```python
from build123d import *

# Parameters (mm, degrees)
BOSS_EXTRUDE1_DEPTH = 12.7
SKETCH2_R           = 2.032
SKETCH2_R_2         = 3.96875
CUT_EXTRUDE1_DEPTH  = 93.361945119
SKETCH3_R           = 1.1303
CUT_EXTRUDE2_DEPTH  = 4.7625


with BuildPart() as part:
    # Sketch1 → Boss-Extrude1 (new body)
    with BuildSketch(Plane(origin=(0, 0, 0), x_dir=(1, 0, 0), z_dir=(0, 1, 0))):
        Polygon((16.51, 0), (4.7625, 0), (4.7625, 4.7625), (-4.7625, 4.7625), (-4.7625, 0), (-16.51, 0), (-16.51, -26.9875), (-38.1, -26.9875), (-38.1, -33.3375), (-33.3375, -33.3375), (-33.3375, -50.8), (-38.1, -50.8), (-38.1, -57.15), (38.1, -57.15), (38.1, -50.8), (33.3375, -50.8), (33.3375, -33.3375), (38.1, -33.3375), (38.1, -26.9875), (16.51, -26.9875), align=None)
    extrude(amount=BOSS_EXTRUDE1_DEPTH)

    # Sketch2 → Cut-Extrude1 (cut, through all)
    with BuildSketch(Plane(origin=(33.3375, 0, 0), x_dir=(0, 0, -1), z_dir=(1, 0, 0))):
        with Locations((-42.06875, 6.35)):
            Circle(SKETCH2_R)
        with Locations((-12.7, 6.35)):
            Circle(SKETCH2_R_2)
    extrude(amount=-CUT_EXTRUDE1_DEPTH, mode=Mode.SUBTRACT)

    # Sketch3 → Cut-Extrude2 (cut)
    with BuildSketch(Plane(origin=(0, 0, 0), x_dir=(-1, 0, 0), z_dir=(0, 0, -1))):
        with Locations((-10.16, 6.35)):
            Circle(SKETCH3_R)
        with Locations((10.16, 6.35)):
            Circle(SKETCH3_R)
    extrude(amount=-CUT_EXTRUDE2_DEPTH, mode=Mode.SUBTRACT)


solid = part.part
```
The model under review builds one solid part; all positions refer to its coordinate system, in mm. A direction names the side the tool comes from. Round coordinates to 2 decimals unless told otherwise and drop trailing zeros. Loops run counter-clockwise (first coordinate to the right, second up) from the corner with the lowest first, then second, coordinate; pieces in that order, holes last. Notation, with made-up numbers: (48, 41) -> (96, 41) arc R32 ccw to (96, 68) -> close; hole circle Ø5 at (-6, 20). An arc over 180 degrees is marked (long way). Answer as a JSON object with one key per item and string values. Group by question number.
1) We need section B-B on x = 13. Write out the cut boundary in (y, z), then the cut area to 3 significant figures.
2) We need section A-A on z = 12.7. Write out the cut boundary in (x, y), then the cut area to 3 significant figures.
3) We need section D-D on y = 11.75. Write out the cut boundary in (x, z).
4) For pin 1 Ø1.1 at (x, y) = (10.5, 6.5) entering from -Z; pin 2 Ø6.5 at (x, y) = (-30.5, 8) entering from -Z; pin 3 Ø5 at (y, z) = (7.5, 12.5) entering from +X; pin 4 Ø3.5 at (x, y) = (9.5, 4.5) entering from -Z, all flat-tipped, find the tip position at first contact; note any pin that passes through.
5) For faces 1 (the face through (33.338, 8, 44)), 2 (the face through (12, 6, 0)), 3 (the face through (-36, 6, 33.338)), 4 (the face through (-4.762, 6, -2)), list the 3-axis set-ups (+Z, -Z, +X, -X, +Y, -Y) from which the entire face can be reached by the end or side of a thin tool; tool diameter is ignored.
6) For line 1 (Y direction, x = 10.16, z = 1.95); line 2 (Z direction, x = 34.5, y = 1.25); line 3 (Z direction, x = -6.5, y = 1.25), list the stretches that pass through material, from the lowest coordinate up. Write a range as [from, to].
7) We need section C-C on x = 29.5. Write out the cut boundary in (y, z).
8) Mouldability with a two-part tool opening along X and no side actions: class faces 5 (the face through (-9.327, 7.114, 2.348)), 6 (the face through (-33.338, 8, 40)), 7 (the face through (0.5, 6.4, 44.1)) as released by +X, released by -X, zero draft, split by the parting line, or undercut.
Result set:
{
 "1": {"outline": "(0, 0) -> (12.7, 0) -> (12.7, 57.15) -> (0, 57.15) -> close; hole circle Ø7.94 at (6.35, 12.7); hole circle Ø4.06 at (6.35, 42.07)", "area": "663 mm²"},
 "2": {"outline": "(-16.51, 0) -> (16.51, 0) -> (16.51, 2.38) -> (-16.51, 2.38) -> close; (-16.51, 10.32) -> (16.51, 10.32) -> (16.51, 12.7) -> (-16.51, 12.7) -> close", "area": "157 mm²"},
 "3": {"outline": "(-38.1, 26.99) -> (-16.51, 26.99) -> (-16.51, 0) -> (-4.76, 0) -> (-4.76, -4.76) -> (4.76, -4.76) -> (4.76, 0) -> (16.51, 0) -> (16.51, 26.99) -> (38.1, 26.99) -> (38.1, 33.34) -> (33.34, 33.34) -> (33.34, 50.8) -> (38.1, 50.8) -> (38.1, 57.15) -> (-38.1, 57.15) -> (-38.1, 50.8) -> (-33.34, 50.8) -> (-33.34, 33.34) -> (-38.1, 33.34) -> close"},
 "4": {"pin 1": "z = 4.76", "pin 2": "z = 26.99", "pin 3": "through", "pin 4": "z = 0"},
 "5": {"face 1": "+X, +Y, -Y", "face 2": "-Z, +X, +Y, -Y", "face 3": "-X, +Y, -Y", "face 4": "-Z, -X, +Y, -Y"},
 "6": {"line 1": "[0, 5.22], [7.48, 12.7]", "line 2": "[26.99, 33.34], [50.8, 57.15]", "line 3": "[0, 57.15]"},
 "7": {"outline": "(0, 26.99) -> (12.7, 26.99) -> (12.7, 57.15) -> (0, 57.15) -> close; hole circle Ø4.06 at (6.35, 42.07)"},
 "8": {"face 5": "undercut", "face 6": "released by -X", "face 7": "zero draft"}
}
